For this review, use the dimensioned drawing (mm, ordinates from the lowest corner) and the shaded views. Give positions to 0.01 mm unless a question says otherwise; leave off trailing zeros. Write each loop counter-clockwise with the first axis right and the second up, starting at its lowest first coordinate (ties: lowest second). Pieces come first, ordered by that corner, then holes. Notation, with made-up numbers: M -4,86.5 L 39,86.5 A22 cw 39,105.5 Z; hole C -14.75,7.5 d9. An arc over 180 degrees is marked long. One line per item, written item: value. Start each with the question number.
Item 1: Consider section D-D, the plane y = 6.75. Write out the cut boundary in (x, z).
Item 2: Consider section A-A, the plane z = 3.5. Write out the cut boundary in (x, y).
Item 3: To check wall thickness, follow probe 1 along Y at (x, z) = (3.75, 3.5); probe 2 along Y at (x, z) = (5.5, 5); probe 3 along Z at (x, y) = (6.75, 3.25). State the ranges of each line that lie inside material, in increasing order.
Item 4: Consider section C-C, the plane x = 7. Write out the cut boundary in (y, z), and give its area (3 significant figures).
Item 5: Mouldability with a two-part tool opening along Z and no side actions: class the marked faces 1, 2 and 3 as released by +Z, released by -Z, zero draft, split by the parting line, or undercut.
Item 6: Clearance check with flat-ended pins moving along their axes: pin 1 Ø1 at (x, z) = (5.5, 1.5) entering from +Y; pin 2 Ø1.5 at (x, z) = (1.5, 4.5) entering from +Y. State where each tip first meets the part, or that it passes through.
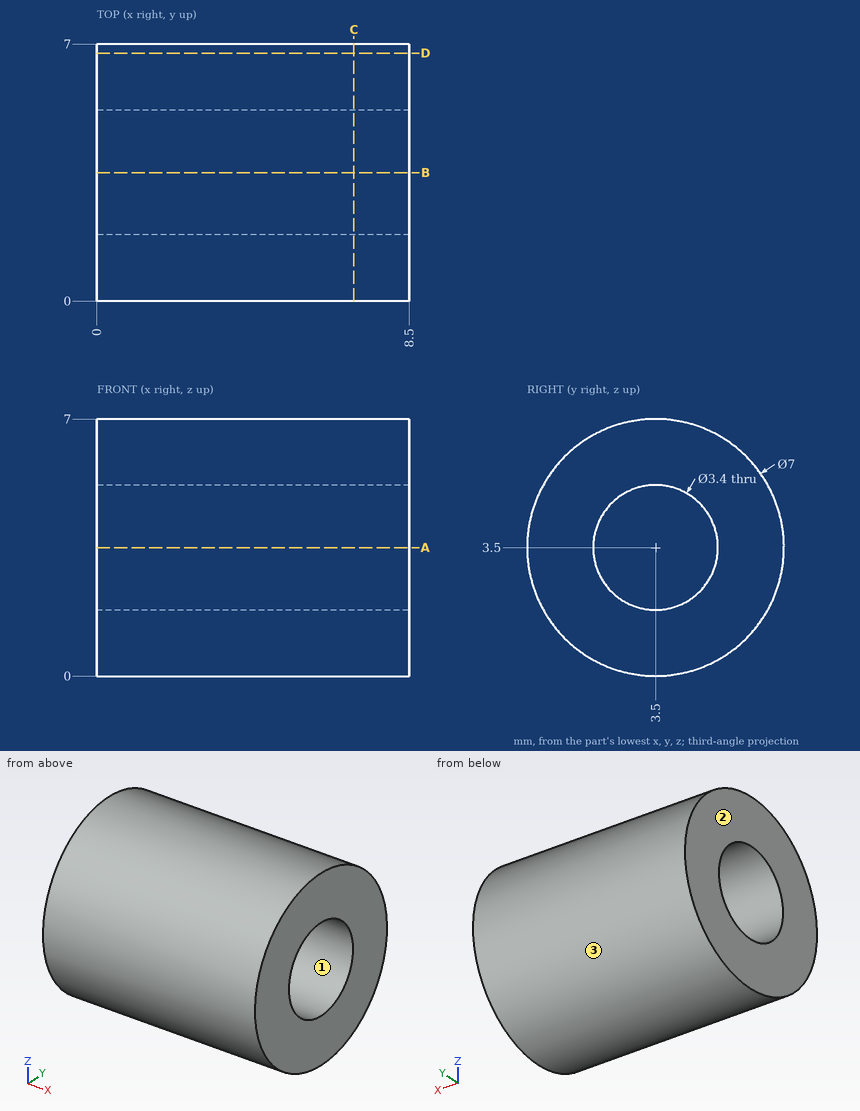
Model answer:
1. outline: M 0,2.2 L 8.5,2.2 L 8.5,4.8 L 0,4.8 Z
2. outline: M 0,0 L 8.5,0 L 8.5,1.8 L 0,1.8 Z; M 0,5.2 L 8.5,5.2 L 8.5,7 L 0,7 Z
3. probe 1: y = 0 to 1.8, 5.2 to 7
3. probe 2: y = 0.34 to 2.7, 4.3 to 6.66
3. probe 3: z = 0.01 to 1.82, 5.18 to 6.99
4. outline: C 3.5,3.5 d7; hole C 3.5,3.5 d3.4
4. area: 29.4 mm2
5. face 1: undercut
5. face 2: zero draft
5. face 3: split by the parting line
6. pin 1: stops at y = 6.66
6. pin 2: stops at y = 6.99
